Can you work these out from the model? Positions are in its coordinate system, mm. Round coordinates to 2 decimals unless told otherwise and drop trailing zeros. Loops run counter-clockwise (first coordinate to the right, second up) from the corner with the lowest first, then second, coordinate; pieces in that order, holes last. Notation, with made-up numbers: (6, 52) -> (39, 52) arc R30 cw to (39, 86) -> close; hole circle Ø6 at (80, -34.75). An arc over 180 degrees is marked (long way). Use a Markdown table: item, result.
Autodesk Inventor part; units mm, degrees
ref_plane "YZ Plane" through (0, 0, 0) normal (1, 0, 0) x (0, 1, 0)
ref_plane "XZ Plane" through (0, 0, 0) normal (0, 1, 0) x (-1, 0, 0)
ref_plane "XY Plane" through (0, 0, 0) normal (0, 0, 1) x (1, 0, 0)
sketch "Sketch1" plane through (0, 0, 0) normal (0, 0, 1) x (1, 0, 0)
  line L0 (-9.525, 0) -> (9.525, 0)
  line L1 (9.525, 0) -> (9.525, 15.875)
  line L2 (-9.525, 0) -> (-9.525, 15.875)
  arc A0 (9.525, 15.875) -> (-9.525, 15.875) centre (0, 15.875) ccw
  point P0 (0, 0)
  dimension "d0" = 19.05
  dimension "d1" = 9.525
  dimension "d2" = 9.525
  dimension "d3" = 15.875
extrude "Extrusion1" add sketch "Sketch1" along normal blind 12.7
hole "Hole1" at (0, 22.225, 12.7) direction (0, 0, -1) diameter 2.2606 depth 6.35
properties part number "Rudder_Bracket"
1. I want a section at D-D (y = 19.25). Please give me the cut outline in (x, z).
Answer sheet:
| item | result |
|---|---|
| outline | (-8.91, 0) -> (8.91, 0) -> (8.91, 12.7) -> (-8.91, 12.7) -> close |
2. I want a section at A-A (z = 7). Please give me the cut outline in (x, y) (3 decimals), plus the area to 3 significant figures.
Answer sheet:
| item | result |
|---|---|
| outline | (-9.525, 0) -> (9.525, 0) -> (9.525, 15.875) arc R9.525 ccw to (-9.525, 15.875) -> close; hole circle Ø2.261 at (0, 22.225) |
| area | 441 mm² |
3. If we mould it in two halves opening along X, with no side actions, what happens to faces 1 (the cylindrical face through (-0.05, 23.354, 9.481)), 2 (the flat face through (0, 22, 6.35)), 3 (the cylindrical face through (-0.209, 25.398, 6.261)), 4 (the flat face through (9.525, 8, 6))? For each: +X half, -X half, draft (parallel to the pull), parting line (faces both ways), or undercut.
Answer sheet:
| item | result |
|---|---|
| face 1 | undercut |
| face 2 | undercut |
| face 3 | parting line |
| face 4 | +X half |
4. I need wall thicknesses on line 1 (Y direction, x = 0, z = 10.25); line 2 (X direction, y = 22.75, z = 8); line 3 (X direction, y = 21.25, z = 9.75). Which ranges of each line are inside material? Lowest first, please.
Answer sheet:
| item | result |
|---|---|
| line 1 | y = 0 to 21.09, 23.36 to 25.4 |
| line 2 | x = -6.59 to -1, 1 to 6.59 |
| line 3 | x = -7.86 to -0.57, 0.57 to 7.86 |
5. Will these pins go through, and if not, where does the flat tip stop? pin 1 Ø5 at (x, y) = (0, 16.5) entering from -Z; pin 2 Ø1 at (x, z) = (-5.5, 4) entering from +Y.
Answer sheet:
| item | result |
|---|---|
| pin 1 | stops at z = 0 |
| pin 2 | stops at y = 23.98 |
6. I want a section at B-B (x = 0). Please give me the cut outline in (y, z), plus the area to 3 significant figures.
Answer sheet:
| item | result |
|---|---|
| outline | (0, 0) -> (25.4, 0) -> (25.4, 12.7) -> (23.36, 12.7) -> (23.36, 6.35) -> (21.09, 6.35) -> (21.09, 12.7) -> (0, 12.7) -> close |
| area | 308 mm² |
7. I want a section at C-C (z = 1.5). Please give me the cut outline in (x, y) (3 decimals), plus the area to 3 significant figures.
Answer sheet:
| item | result |
|---|---|
| outline | (-9.525, 0) -> (9.525, 0) -> (9.525, 15.875) arc R9.525 ccw to (-9.525, 15.875) -> close |
| area | 445 mm² |
